Autodesk Inventor part; units mm, degrees
ref_plane "YZ Plane" through (0, 0, 0) normal (1, 0, 0) x (0, 1, 0)
ref_plane "XZ Plane" through (0, 0, 0) normal (0, 1, 0) x (-1, 0, 0)
ref_plane "XY Plane" through (0, 0, 0) normal (0, 0, 1) x (1, 0, 0)
sketch "Sketch1" plane through (0, 0, 0) normal (0, 0, 1) x (1, 0, 0)
  line L0 (-6.35, -3.6662) -> (-6.35, 3.6662)
  line L1 (-6.35, 3.6662) -> (0, 7.3323)
  line L2 (0, 7.3323) -> (6.35, 3.6662)
  line L3 (6.35, 3.6662) -> (6.35, -3.6662)
  line L4 (6.35, -3.6662) -> (0, -7.3323)
  line L5 (0, -7.3323) -> (-6.35, -3.6662)
  point P0 (0, 0)
  point P1 (0, 0)
  dimension "Size" = 12.7
extrude "Extrusion1" add sketch "Sketch1" along normal mid plane 184.15
sketch "Sketch3" plane through (0, 0, 92.075) normal (0, 0, 1) x (1, 0, 0)
  line L0 (-6.35, 3.6662) -> (0, 7.3323) construction
  line L1 (0, 7.3323) -> (6.35, 3.6662) construction
  line L2 (6.35, 3.6662) -> (6.35, -3.6662) construction
  line L3 (6.35, -3.6662) -> (0, -7.3323) construction
  line L4 (0, -7.3323) -> (-6.35, -3.6662) construction
  line L5 (-6.35, -3.6662) -> (-6.35, 3.6662) construction
  point P0 (0, 0)
hole "Hole1" at (0, 0, 92.075) direction (0, 0, -1) diameter 5.1054 end through all
sketch "Sketch4" plane through (0, 0, 92.075) normal (0, 0, 1) x (1, 0, 0)
  circle A0 centre (0, 0) radius 2.5527 construction
  line L0 (-6.35, 3.6662) -> (0, 7.3323) construction
  line L1 (0, 7.3323) -> (6.35, 3.6662) construction
  line L2 (6.35, 3.6662) -> (6.35, -3.6662) construction
  line L3 (6.35, -3.6662) -> (0, -7.3323) construction
  line L4 (0, -7.3323) -> (-6.35, -3.6662) construction
  line L5 (-6.35, -3.6662) -> (-6.35, 3.6662) construction
  circle A1 centre (0, 0) radius 6.8771
  circle A2 centre (0, 0) radius 8.89
  dimension "thunder" = 13.7541
  dimension "d16" = 17.78
extrude "Extrusion3" cut sketch "Sketch4" against normal through all
equation "\"bearing\" = 25.4"
properties part number "GP5-024" material "Aluminum 6061"
Can you work these out from the model? Positions are in its coordinate system, mm. Give positions to 0.01 mm unless a question says otherwise; leave off trailing zeros. Loops run counter-clockwise (first coordinate to the right, second up) from the corner with the lowest first, then second, coordinate; pieces in that order, holes last. Notation, with made-up numbers: (-19.5, 73.5) -> (-11.5, 73.5) arc R18 cw to (-11.5, 79.5) -> close; hole circle Ø1 at (-5.5, 51). An arc over 180 degrees is marked (long way). Write item = value, one per line.
1) Will these pins go through, and if not, where does the flat tip stop? pin 1 (1.5 mm diameter, centred on x = 2, z = 62.5, fed in from +Y); pin 2 (4 mm diameter, centred on x = 3, z = 26.5, fed in from +Y).
Check result:
pin_1 = 6.61
pin_2 = 6.75
2) Suppose I cut it at A-A on z = -48.5. Write out the boundary of the cut face in (x, y), then the cut area to 3 significant figures.
Check result:
outline = (-6.35, -2.64) arc R6.88 ccw to (-5.46, -4.18) -> (-0.89, -6.82) arc R6.88 ccw to (0.89, -6.82) -> (5.46, -4.18) arc R6.88 ccw to (6.35, -2.64) -> (6.35, 2.64) arc R6.88 ccw to (5.46, 4.18) -> (0.89, 6.82) arc R6.88 ccw to (-0.89, 6.82) -> (-5.46, 4.18) arc R6.88 ccw to (-6.35, 2.64) -> close; hole circle Ø5.11 at (0, 0)
area = 117 mm2
3) Thinking about a two-plate mould opening in X: for faces 1 (the cylindrical face through (-0.767, -2.435, -1.289)), 2 (the flat face through (-6.35, 0, -1)), 3 (the flat face through (3.21, -5.48, -1.29)), 4 (the flat face through (-3, 0, 92.075)), which applies, released by +X, released by -X, zero draft, split by the parting line, or undercut?
Check result:
face_1 = undercut
face_2 = released by -X
face_3 = released by +X
face_4 = zero draft
4) I need wall thicknesses on L1, parallel to X at y = 0, z = 16; L2, parallel to Y at x = 0, z = 45.5; L3, parallel to Y at x = -0.5, z = 53. Which ranges of each line are inside material? Lowest first, please. Write a range as from..to.
Check result:
L1 = -6.35..-2.55, 2.55..6.35
L2 = -6.88..-2.55, 2.55..6.88
L3 = -6.86..-2.5, 2.5..6.86
5) Suppose I cut it at B-B on y = 0. Write out the boundary of the cut face in (x, z) (3 decimals).
Check result:
outline = (-6.35, -92.075) -> (-2.553, -92.075) -> (-2.553, 92.075) -> (-6.35, 92.075) -> close; (2.553, -92.075) -> (6.35, -92.075) -> (6.35, 92.075) -> (2.553, 92.075) -> close
